from build123d import *

# Parameters (mm, degrees)
SKETCH2_W         = 381
SKETCH2_H         = 381
SKETCH2_R         = 3.3782
BOLT_HOLES_DEPTH  = 19.05
SKETCH3_R         = 12.5
COUNTERBORE_DEPTH = 12.7
SKETCH4_W         = 203.708
SKETCH4_H         = 203.708
AL_POCKET_DEPTH   = 3.175
RELIEF_DEPTH      = 6.35


with BuildPart() as part:
    # Sketch2 → Bolt Holes (new body)
    with BuildSketch(Plane(origin=(0, 0, 0), x_dir=(1, 0, 0), z_dir=(0, 1, 0))):
        Rectangle(SKETCH2_W, SKETCH2_H)
        with Locations(Location((0, 0, 0), (0, 0, 90))):
            Circle(SKETCH2_R, mode=Mode.SUBTRACT)
        with Locations(Location((0, 50.8, 0), (0, 0, 90))):
            Circle(SKETCH2_R, mode=Mode.SUBTRACT)
        with Locations(Location((0, 101.6, 0), (0, 0, 90))):
            Circle(SKETCH2_R, mode=Mode.SUBTRACT)
        with Locations(Location((0, 152.4, 0), (0, 0, 90))):
            Circle(SKETCH2_R, mode=Mode.SUBTRACT)
        with Locations(Location((0, -50.8, 0), (0, 0, 90))):
            Circle(SKETCH2_R, mode=Mode.SUBTRACT)
        with Locations(Location((0, -101.6, 0), (0, 0, 90))):
            Circle(SKETCH2_R, mode=Mode.SUBTRACT)
        with Locations(Location((0, -152.4, 0), (0, 0, 90))):
            Circle(SKETCH2_R, mode=Mode.SUBTRACT)
    extrude(amount=BOLT_HOLES_DEPTH)

    # Sketch3 → Counterbore (cut)
    with BuildSketch(Plane(origin=(0, 19.05, 0), x_dir=(1, 0, 0), z_dir=(0, 1, 0))):
        with Locations(Location((0, -50.8, 0), (0, 0, 270))):
            Circle(SKETCH3_R)
        with Locations(Location((0, 0, 0), (0, 0, 270))):
            Circle(SKETCH3_R)
        with Locations(Location((0, -101.6, 0), (0, 0, 270))):
            Circle(SKETCH3_R)
        with Locations(Location((0, 50.8, 0), (0, 0, 270))):
            Circle(SKETCH3_R)
        with Locations(Location((0, 101.6, 0), (0, 0, 270))):
            Circle(SKETCH3_R)
        with Locations(Location((0, 152.4, 0), (0, 0, 270))):
            Circle(SKETCH3_R)
        with Locations(Location((0, -152.4, 0), (0, 0, 270))):
            Circle(SKETCH3_R)
    extrude(amount=-COUNTERBORE_DEPTH, mode=Mode.SUBTRACT)

    # Sketch4 → al_pocket (cut)
    with BuildSketch(Plane(origin=(0, 19.05, 0), x_dir=(1, 0, 0), z_dir=(0, 1, 0))):
        with Locations((-63.246, -63.246)):
            Rectangle(SKETCH4_W, SKETCH4_H)
    extrude(amount=-AL_POCKET_DEPTH, mode=Mode.SUBTRACT)

    # Sketch5 → Relief (cut)
    with BuildSketch(Plane(origin=(0, 19.05, 0), x_dir=(1, 0, 0), z_dir=(0, 1, 0))):
        with BuildLine():
            Line((-174.625, 38.608), (-155.575, 38.608))
            ThreePointArc((-155.575, 38.608), (-149.225, 32.258), (-155.575, 25.908))
            Line((-155.575, 25.908), (-174.625, 25.908))
            ThreePointArc((-174.625, 25.908), (-180.975, 32.258), (-174.625, 38.608))
        make_face()
        with BuildLine():
            Line((-174.625, -152.4), (-155.575, -152.4))
            ThreePointArc((-155.575, -152.4), (-149.225, -158.75), (-155.575, -165.1))
            Line((-155.575, -165.1), (-174.625, -165.1))
            ThreePointArc((-174.625, -165.1), (-180.975, -158.75), (-174.625, -152.4))
        make_face()
        with BuildLine():
            Line((-174.625, -56.642), (-155.575, -56.642))
            ThreePointArc((-155.575, -56.642), (-149.225, -62.992), (-155.575, -69.342))
            Line((-155.575, -69.342), (-174.625, -69.342))
            ThreePointArc((-174.625, -69.342), (-180.975, -62.992), (-174.625, -56.642))
        make_face()
        with BuildLine():
            Line((29.083, 38.608), (48.133, 38.608))
            ThreePointArc((48.133, 38.608), (54.483, 32.258), (48.133, 25.908))
            Line((48.133, 25.908), (29.083, 25.908))
            ThreePointArc((29.083, 25.908), (22.733, 32.258), (29.083, 38.608))
        make_face()
        with BuildLine():
            Line((29.083, -152.4), (48.133, -152.4))
            ThreePointArc((48.133, -152.4), (54.483, -158.75), (48.133, -165.1))
            Line((48.133, -165.1), (29.083, -165.1))
            ThreePointArc((29.083, -165.1), (22.733, -158.75), (29.083, -152.4))
        make_face()
        with BuildLine():
            Line((29.083, -56.642), (48.133, -56.642))
            ThreePointArc((48.133, -56.642), (54.483, -62.992), (48.133, -69.342))
            Line((48.133, -69.342), (29.083, -69.342))
            ThreePointArc((29.083, -69.342), (22.733, -62.992), (29.083, -56.642))
        make_face()
    extrude(amount=-RELIEF_DEPTH, mode=Mode.SUBTRACT)


solid = part.part
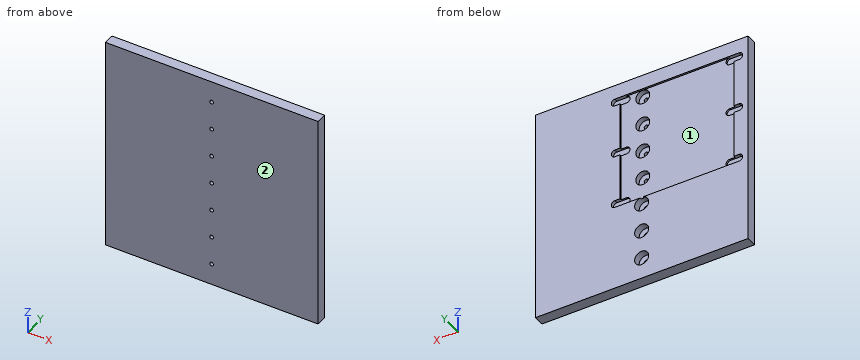
Could you check a few things on this model? Use its own coordinates, in mm. Face numbers are marked on the shaded views. Round coordinates to 2 decimals unless told otherwise and drop trailing zeros. Write each loop counter-clockwise with the first axis right and the second up, starting at its lowest first coordinate (ties: lowest second). Pieces come first, ordered by that corner, then holes. Notation, with made-up numbers: (15.25, 12.25) - (48.25, 12.25) arc R26 ccw to (48.25, 28.25) - close; hole circle Ø10 at (-8.75, -36). An arc over 180 degrees is marked (long way). Put each result on its own line as item: value. Start each with the question number.
(1) I need wall thicknesses on probe 1 along Z at (x, y) = (43, 15.5); probe 2 along X at (y, z) = (15.25, -50.8); probe 3 along X at (y, z) = (2, 0). Which ranges of each line are inside material? Lowest first, please.
(2) Thinking about a two-plate mould opening in X: for the marked faces 1 and 2, which applies, released by +X, released by -X, zero draft, split by the parting line, or undercut?
(3) I want a section at A-A, the plane x = -140. Please give me the cut outline in (y, z) (3 decimals), plus the area to 3 significant figures.
(4) Will these pins go through, and if not, where does the flat tip stop? pin 1 (6.5 mm diameter, centred on x = -164, z = 158, fed in from +Y); pin 2 (12 mm diameter, centred on x = -120, z = 128, fed in from +Y) (3 decimals).
Here are the results:
1. probe 1: z = -190.5 to -38.61, -25.91 to 56.64, 69.34 to 152.4, 165.1 to 190.5
1. probe 2: x = -190.5 to -12.5, 12.5 to 190.5
1. probe 3: x = -190.5 to -3.38, 3.38 to 190.5
2. face 1: undercut
2. face 2: zero draft
3. outline: (0, -190.5) - (19.05, -190.5) - (19.05, -38.608) - (15.875, -38.608) - (15.875, 165.1) - (19.05, 165.1) - (19.05, 190.5) - (0, 190.5) - close
3. area: 6,610 mm^2
4. pin 1: stops at y = 12.7
4. pin 2: stops at y = 15.875
